```python
from build123d import *

# Parameters (mm, degrees)
F0_W     = 30
F0_H     = 10
F0_R     = 2.75
F1_DEPTH = 4
F2_DEPTH = 8
F3_START = 2
F0_R_2   = 1.9
F3_DEPTH = 6
F4_R     = 1


with BuildPart() as f1:
    # F0 (on Top) → F1 (new body)
    with BuildSketch(Plane.XY):
        with Locations((15, 15)):
            Rectangle(F0_W, F0_H)
        with Locations((5, 15)):
            Circle(F0_R, mode=Mode.SUBTRACT)
        with Locations((25, 15)):
            Circle(F0_R, mode=Mode.SUBTRACT)
    extrude(amount=F1_DEPTH)

    # F0 (on Top) → F2 (join)
    with BuildSketch(Plane.XY):
        with Locations((15, 5)):
            Rectangle(F0_W, F0_H)
        Polygon((3.95, 2.3153212483), (2.4, 5), (3.95, 7.6846787517), (7.05, 7.6846787517), (8.6, 5), (7.05, 2.3153212483), align=None, mode=Mode.SUBTRACT)
        Polygon((22.95, 2.3153212483), (21.4, 5), (22.95, 7.6846787517), (26.05, 7.6846787517), (27.6, 5), (26.05, 2.3153212483), align=None, mode=Mode.SUBTRACT)
    extrude(amount=F2_DEPTH)

    # F0 (on Top) → F3 (join)
    with BuildSketch(Plane.XY.offset(F3_START)):
        Polygon((3.95, 7.6846787517), (2.4, 5), (3.95, 2.3153212483), (7.05, 2.3153212483), (8.6, 5), (7.05, 7.6846787517), align=None)
        with Locations((5.5, 5)):
            Circle(F0_R_2, mode=Mode.SUBTRACT)
        Polygon((22.95, 7.6846787517), (21.4, 5), (22.95, 2.3153212483), (26.05, 2.3153212483), (27.6, 5), (26.05, 7.6846787517), align=None)
        with Locations((24.5, 5)):
            Circle(F0_R_2, mode=Mode.SUBTRACT)
    extrude(amount=F3_DEPTH)

    # F4
    f4_edges = [f1.edges().sort_by_distance(p)[0] for p in [
        (0, 5, 8),
        (15, 0, 8),
        (30, 5, 8),
        (15, 10, 8),
        (15, 10, 4),
        (15, 20, 4),
        (0, 15, 4),
        (30, 15, 4),
        (0, 10, 6),
        (30, 10, 6),
        (0, 0, 4),
        (0, 10, 0),
        (0, 20, 2),
        (15, 20, 0),
        (30, 20, 2),
        (30, 10, 0),
        (30, 0, 4),
        (15, 0, 0),
    ]]
    fillet(f4_edges, radius=F4_R)


solid = f1.part
```
Source: CAD feature listing. Evaluate the final solid. Frame: model axes, mm. A direction names the side the tool comes from. Give positions to 0.01 mm unless a question says otherwise; leave off trailing zeros. Order: outer loops, then holes, each group sorted by start corner. A loop starts at its lowest first (then second) coordinate and runs counter-clockwise, first axis right, second up.
(1) Material intervals for line 1 along Y through (x, z) = (25, 1.35); line 2 along Y through (x, z) = (25, 2.95); line 3 along X through (y, z) = (2.75, 1), sorted ascending.
(2) Section query D-D (y = 11.5). Return the cut outline in (x, z), plus the area to 3 significant figures.
(3) Pull-direction query (Y, two-part tool) for faces 4 (the face through (0, 8, 3)), 5 (the face through (25, 2.315, 1)), 6 (the face through (15.196, 19.699, 0.285)); classes: +Y half, -Y half, draft (parallel to the pull), parting line (faces both ways), or undercut.
(4) Section query C-C (x = 12). Return the cut outline in (y, z), plus the area to 3 significant figures.
(5) Section query B-B (x = 24.5). Return the cut outline in (y, z), plus the area to 3 significant figures.
(6) Contact query for flat-ended pins moving along their axis: P1, Ø2.5, axis at x = 7, y = 5, coming from the -Z side; P2, Ø4, axis at x = 20, y = 14.5, coming from the +Z side; P3, Ø2, axis at x = 9.5, z = 5.5, coming from the +Y side. Output: stop coordinate, or through.
(7) Section query A-A (y = 15). Return the cut outline in (x, z).
(8) Access query for faces 1 (the face through (6, 7, 2)), 2 (the face through (29.715, 15.056, 3.699)), 3 (the face through (15, 10, 6)). Directions: +Z, -Z, +X, -X, +Y, -Y. A direction counts if a zero-diameter tool reaches every point of the face in a straight line with its end or side. Return the directions, or none.
Outcome:
1. line 1: y = 0 to 2.32, 7.68 to 12.25, 17.75 to 20
1. line 2: y = 0 to 3.17, 6.83 to 12.25, 17.75 to 20
1. line 3: x = 0 to 3.7, 7.3 to 22.7, 26.3 to 30
2. outline: (0, 1) arc R1 ccw to (1, 0) - (29, 0) arc R1 ccw to (30, 1) - (30, 3) arc R1 ccw to (29, 4) - (1, 4) arc R1 ccw to (0, 3) - close
2. area: 119 mm2
3. face 4: draft
3. face 5: undercut
3. face 6: +Y half
4. outline: (0, 1) arc R1 ccw to (1, 0) - (19, 0) arc R1 ccw to (20, 1) - (20, 3) arc R1 ccw to (19, 4) - (11, 4) arc R1 cw to (10, 5) - (10, 7) arc R1 ccw to (9, 8) - (1, 8) arc R1 ccw to (0, 7) - close
4. area: 119 mm2
5. outline: (0, 1) arc R1 ccw to (1, 0) - (2.32, 0) - (2.32, 2) - (3.1, 2) - (3.1, 8) - (1, 8) arc R1 ccw to (0, 7) - close; (6.9, 2) - (7.68, 2) - (7.68, 0) - (12.3, 0) - (12.3, 4) - (11, 4) arc R1 cw to (10, 5) - (10, 7) arc R1 ccw to (9, 8) - (6.9, 8) - close; (17.7, 0) - (19, 0) arc R1 ccw to (20, 1) - (20, 3) arc R1 ccw to (19, 4) - (17.7, 4) - close
5. area: 64.0 mm2
6. P1: stops at z = 2
6. P2: stops at z = 4
6. P3: stops at y = 10.13
7. outline: (0, 1) arc R1 ccw to (1, 0) - (2.25, 0) - (2.25, 4) - (1, 4) arc R1 ccw to (0, 3) - close; (7.75, 0) - (22.25, 0) - (22.25, 4) - (7.75, 4) - close; (27.75, 0) - (29, 0) arc R1 ccw to (30, 1) - (30, 3) arc R1 ccw to (29, 4) - (27.75, 4) - close
8. face 1: -Z
8. face 2: +Z, +X, +Y
8. face 3: +Z, +X, -X, +Y
